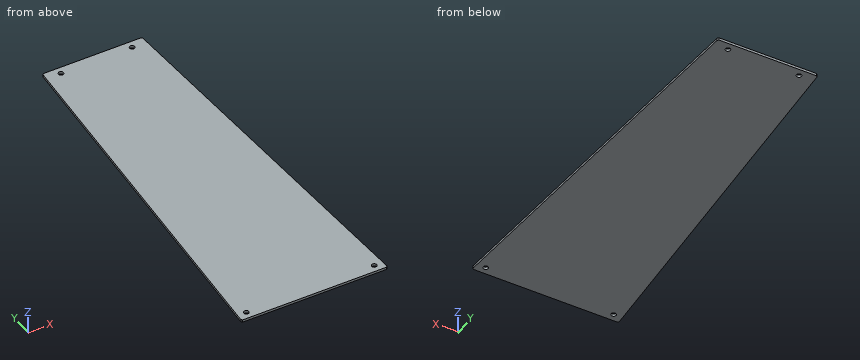
Autodesk Inventor part; units mm, degrees
ref_plane "YZ Plane" through (0, 0, 0) normal (1, 0, 0) x (0, 1, 0)
ref_plane "XZ Plane" through (0, 0, 0) normal (0, 1, 0) x (-1, 0, 0)
ref_plane "XY Plane" through (0, 0, 0) normal (0, 0, 1) x (1, 0, 0)
ref_plane "Work Plane1" through (0, 0, 0) normal (0, 0, 1) x (1, 0, 0)
sketch "Sketch1" plane through (0, 0, 0) normal (0, 0, 1) x (1, 0, 0)
  line L0 (143.1602, 7.9375) -> (124.1349, 317.827) construction
  line L1 (145.6, 317.827) -> (20, 317.827) construction
  line L2 (41.4651, 317.827) -> (22.4398, 7.9375) construction
  line L3 (165.6, 7.9375) -> (0, 7.9375) construction
  line L4 (41.4651, 317.827) -> (124.1349, 317.827)
  line L5 (124.1349, 317.827) -> (143.1602, 7.9375)
  line L6 (143.1602, 7.9375) -> (22.4398, 7.9375)
  line L7 (22.4398, 7.9375) -> (41.4651, 317.827)
  line L8 (42.4056, 316.827) -> (123.1944, 316.827)
  line L9 (123.1944, 316.827) -> (142.097, 8.9375)
  line L10 (142.097, 8.9375) -> (23.503, 8.9375)
  line L11 (23.503, 8.9375) -> (42.4056, 316.827)
  point P0 (0, 0)
  dimension "d2" = 1
extrude "Extrusion1" add sketch "Sketch1" along normal blind 2 contours L8 L9 L10 L11
chamfer "Chamfer1" distance 1 angle 45 4 edges at (123.1944, 316.827, 1) (42.4056, 316.827, 1) (142.097, 8.9375, 1) (23.503, 8.9375, 1)
sketch "Sketch2" plane through (0, 0, 2) normal (0, 0, 1) x (1, 0, 0)
  line L0 (122.1944, 316.827) -> (43.4056, 316.827) construction
  line L1 (24.503, 8.9375) -> (141.097, 8.9375) construction
  line L2 (43.4056, 316.827) -> (122.1944, 316.827) construction
  line L3 (82.8, 316.827) -> (82.8, 8.9375) construction
  line L4 (141.097, 8.9375) -> (24.503, 8.9375) construction
  point P0 (0, 0)
  point P1 (53.9987, 310.827)
  point P2 (31.008, 14.9375)
  point P3 (111.6013, 310.827)
  point P4 (134.592, 14.9375)
  dimension "d6" = 6
  dimension "d7" = 6
hole "Hole1" at (53.9987, 310.827, 2) at (31.008, 14.9375, 2) at (111.6013, 310.827, 2) at (134.592, 14.9375, 2) direction (0, 0, -1) diameter 4 end through all
properties part number "LowerPlate"
Input: part model. Units: mm. Frame: model coordinates. Round coordinates to 2 decimals unless told otherwise and drop trailing zeros. Write each loop counter-clockwise with the first axis right and the second up, starting at its lowest first coordinate (ties: lowest second). Pieces come first, ordered by that corner, then holes.
1) Contact query for a flat-ended pin moving along its axis: P1, Ø3.5, axis at x = 111.6, y = 310.83, coming from the -Z side. Output: stop coordinate, or through.
2) Ray query, L1, parallel to Y at x = 110.5, z = 1.45; L2, parallel to X at y = 94.5, z = 1.55; L3, parallel to X at y = 143.5, z = 0.8. Return the intervals inside material, ascending.
3) Cut plane A-A (z = 1.7). Return the cut outline in (x, y), then the cut area to 3 significant figures.
4) Cut plane B-B (y = 48). Return the cut outline in (x, z), then the cut area to 3 significant figures.
5) Cut plane C-C (y = 294.5). Return the cut outline in (x, z), then the cut area to 3 significant figures.
Geometry says:
1. P1: passes through
2. L1: y = 8.94 to 309.16, 312.5 to 316.83
2. L2: x = 28.76 to 136.84
2. L3: x = 31.76 to 133.84
3. outline: (23.56, 9.94) - (24.5, 8.94) - (141.1, 8.94) - (142.04, 9.94) - (123.26, 315.83) - (122.19, 316.83) - (43.41, 316.83) - (42.34, 315.83) - close; hole circle Ø4 at (31.01, 14.94); hole circle Ø4 at (54, 310.83); hole circle Ø4 at (111.6, 310.83); hole circle Ø4 at (134.59, 14.94)
3. area: 30,600 mm2
4. outline: (25.9, 0) - (139.7, 0) - (139.7, 2) - (25.9, 2) - close
4. area: 228 mm2
5. outline: (41.03, 0) - (124.57, 0) - (124.57, 2) - (41.03, 2) - close
5. area: 167 mm2
